Work out the finished part from the listing and answer in its coordinate system (mm). A direction names the side the tool comes from. Give positions to 0.01 mm unless a question says otherwise; leave off trailing zeros. One line per item, written item: value.
from build123d import *

# Parameters (mm, degrees)
F0_W           = 8
F0_H           = 50
F1_DEPTH       = 2.5
F2_W           = 15
F2_H           = 1
F2_W_2         = 0.5
F3_DEPTH       = 2
F4_SIZE        = 2.99999
F5_SIZE        = 2
F6_SIZE2       = 0.49999
F6_SIZE        = 0.99999
F7_R           = 1
F9_D           = 3.2
F9_CSINK_D     = 4
F9_CSINK_ANGLE = 82


# Not quite as in the source:
# - a fillet or chamfer is up to 0.001 mm smaller than in the source, because OpenCascade refuses the exact size


with BuildPart() as f1:
    # F0 (on Front) → F1 (new body, symmetric)
    with BuildSketch(Plane.XZ):
        Rectangle(F0_W, F0_H)
        Polygon((7.5, -25), (4, -25), (-4, -25), (-7.5, -25), (-7.5, -28), (7.5, -28), align=None)
    extrude(amount=F1_DEPTH, both=True)

    # F2 (on face) → F3 (cut)
    with BuildSketch(Plane.XZ.offset(2.5)):
        with Locations((0, -27)):
            Rectangle(F2_W, F2_H)
        with Locations((-7.75, -27)):
            Rectangle(F2_W_2, F2_H)
        with Locations((7.75, -27)):
            Rectangle(F2_W_2, F2_H)
    extrude(amount=-F3_DEPTH, mode=Mode.SUBTRACT)

    # F4 (size 3 in the source; OpenCascade refuses exactly that, so slightly less here)
    f4_edges = [f1.edges().sort_by_distance(p)[0] for p in [
        (-7.5, 0, -28),
        (7.5, 0, -28),
    ]]
    chamfer(f4_edges, length=F4_SIZE)

    # F5
    f5_edges = [f1.edges().sort_by_distance(p)[0] for p in [
        (-4, 2.5, 0),
        (4, 2.5, 0),
    ]]
    chamfer(f5_edges, length=F5_SIZE)

    # F6 (size 1 and 0.5 in the source; OpenCascade refuses exactly that, so slightly less here)
    f6_edges = [f1.edges().sort_by_distance(p)[0] for p in [
        (0, -2.5, -27.5),
    ]]
    f6_side = f1.faces().sort_by_distance((0, -1.5, -27.5))[0]
    chamfer(f6_edges, length=F6_SIZE, length2=F6_SIZE2, reference=f6_side)

    # F7
    f7_edges = [f1.edges().sort_by_distance(p)[0] for p in [
        (-5.75, 2.5, -25),
        (5.75, 2.5, -25),
    ]]
    fillet(f7_edges, radius=F7_R)

    # F9 (through all)
    with Locations(Plane(origin=(0, 2.5, 0), x_dir=(-1, 0, 0), z_dir=(0, 1, 0))):
        with Locations((0, 19), (0, 4)):
            CounterSinkHole(F9_D / 2, F9_CSINK_D / 2, counter_sink_angle=F9_CSINK_ANGLE)


solid = f1.part
(1) Which of the six approach directions +Z, -Z, +X, -X, +Y, -Y give full straight-line access (tool end or side, diameter ignored) to faces 1 (the flat face through (-3, 1.5, -0.9)), 2 (the flat face through (0, -2, -26.5)), 3 (the cylindrical face through (4.789, 2.215, -25.301)), 4 (the flat face through (-4, -1, 0)), 5 (the flat face through (4, -1, 0))?
Findings:
face 1: +Z, -X, +Y
face 2: +X, -X, -Y
face 3: +Z, +X, +Y
face 4: +Z, -X, +Y, -Y
face 5: +Z, +X, +Y, -Y
(2) Determine the mould class of faces 6 (the cylindrical face through (-0.208, -0.262, 20.586)), 7 (the flat face through (6, 0, -26.5)), 8 (the flat face through (-6, 0, -26.5)), 9 (the flat face through (0, -2.5, 0)) for opening direction X: pulls with the +X half, pulls with the -X half, needs draft (parallel to the pull), parting line crosses it, or undercut.
Findings:
face 6: undercut
face 7: pulls with the +X half
face 8: pulls with the -X half
face 9: needs draft
(3) Section A-A, the plane x = 0 is taken. Give the number of separate pieces and of enclosed holes in the cut face, then the cut area to 3 significant figures.
Findings:
separate pieces: 3
enclosed holes: 0
area: 230 mm^2
(4) Given P1, Ø0.9, axis at y = -0.5, z = 7.5, coming from the -X side; P2, Ø2.5, axis at y = -1, z = 9.5, coming from the +X side, each flat-ended and moving along its own axis, determine where each tip first touches the part or whether it passes through.
Findings:
P1: stops at x = -4
P2: stops at x = 4
(5) Find the intervals of material crossed by probe 1 along Z at (x, y) = (0, -0.8); probe 2 along Z at (x, y) = (0, 0.45); probe 3 along Z at (x, y) = (-0.5, 0.15), in increasing order. Write a range as from..to.
Findings:
probe 1: z = -28..-27.5, -26.5..2.4, 5.6..17.4, 20.6..25
probe 2: z = -28..2.4, 5.6..17.4, 20.6..25
probe 3: z = -28..2.48, 5.52..17.48, 20.52..25
